Could you check a few things on this model? Use its own coordinates, in mm. Coordinates: 2 decimals unless noted, no trailing zeros.
from build123d import *

# Parameters (mm, degrees)
SKETCH1_W           = 185.999882
SKETCH1_H           = 74.000106
BOSS_EXTRUDE3_DEPTH = 1.5875
CUT_EXTRUDE3_DEPTH  = 2.54


with BuildPart() as part:
    # Sketch1 → Boss-Extrude3 (new body)
    with BuildSketch(Plane(origin=(0, 0, 0), x_dir=(1, 0, 0), z_dir=(0, 1, 0))):
        Rectangle(SKETCH1_W, SKETCH1_H)
    extrude(amount=BOSS_EXTRUDE3_DEPTH)

    # Sketch4 → Cut-Extrude3 (cut)
    with BuildSketch(Plane(origin=(0, 1.5875, 0), x_dir=(1, 0, 0), z_dir=(0, 1, 0))):
        with BuildLine():
            Line((-33.019999998, 0.499998888), (-38.076346482, 0.499998888))
            ThreePointArc((-38.076346482, 0.499998888), (-69.310342417, -8.5e-08), (-38.076346479, -0.499998888))
            Line((-38.076346479, -0.499998888), (-33.019999997, -0.499998888))
            add(Edge.make_bspline(
                [(-33.019999997, -0.499998888), (-32.54632499, -0.569245934), (-31.586035731, -0.710618844), (-29.370983979, -1.038906843), (-27.495063328, -1.325179383), (-25.000131636, -1.708121039), (-22.872397946, -2.043660099), (-20.526372341, -2.417494507), (-18.312405788, -2.778512003), (-16.022726377, -3.157194229), (-13.776510299, -3.536227287), (-10.945442388, -4.021942901), (-6.433516708, -4.814957325), (-1.356746681, -5.744470681), (4.270229912, -6.82483512), (11.013466622, -8.182339851), (16.620878036, -9.365479808), (22.217465189, -10.603163227), (28.231300592, -11.997433679), (33.11855172, -13.176234287), (37.994608625, -14.399821142), (42.858903514, -15.669688211), (47.285116507, -16.866229097), (51.7005538, -18.102139295), (56.104457025, -19.378378553), (59.947265614, -20.531258809), (63.232966999, -21.545846418), (65.965538205, -22.409292492), (68.147965495, -23.110854225), (70.871921061, -24.001687113), (73.589095471, -24.910758606), (76.029944312, -25.746275579), (78.193394279, -26.501694312), (79.81619039, -27.074902775), (81.432049585, -27.651976873), (83.324431409, -28.337781593), (85.465097243, -29.126327671), (87.359843247, -29.836757063), (88.94155129, -30.437597441), (90.322203412, -30.968739967), (91.291423843, -31.343800626), (92.282484454, -31.731855507), (92.741323404, -31.912151608), (92.964000003, -31.999935633)],
                knots=[0.081631279, 0.081631279, 0.081631279, 0.081631279, 0.081631279, 0.096343802, 0.111056325, 0.125768848, 0.140481371, 0.155193894, 0.169906418, 0.184618941, 0.199331464, 0.214043988, 0.228756511, 0.258181558, 0.31703165, 0.346456696, 0.375881743, 0.434731835, 0.464156881, 0.493581928, 0.534357317, 0.563782355, 0.593207404, 0.622632455, 0.652057492, 0.681482549, 0.710907585, 0.725620111, 0.740332636, 0.755045164, 0.769757692, 0.799182725, 0.813895254, 0.821251518, 0.828607782, 0.843320301, 0.858032821, 0.872745338, 0.887457856, 0.894814124, 0.902170393, 0.909526661, 0.91688293, 0.91688293, 0.91688293, 0.91688293, 0.91688293], degree=4))
            Line((92.964000003, -31.999935633), (94.190773048, -31.999935633))
            Line((94.190773048, -31.999935633), (94.190773048, 31.999935633))
            Line((94.190773048, 31.999935633), (92.964000001, 31.999935633))
            add(Edge.make_bspline(
                [(-33.019999998, 0.499998888), (-32.546324991, 0.569245934), (-31.586035733, 0.710618844), (-29.37098398, 1.038906842), (-27.495063329, 1.325179382), (-25.000131637, 1.708121039), (-22.872397948, 2.043660099), (-20.526372343, 2.417494507), (-18.312405789, 2.778512003), (-16.022726379, 3.157194229), (-13.7765103, 3.536227286), (-10.94544239, 4.021942901), (-6.433516709, 4.814957324), (-1.356746682, 5.744470681), (4.27022991, 6.82483512), (11.01346662, 8.182339851), (16.620878035, 9.365479808), (22.217465188, 10.603163227), (28.231300591, 11.997433679), (33.118551718, 13.176234287), (37.994608623, 14.399821142), (42.858903512, 15.669688211), (47.285116506, 16.866229097), (51.700553798, 18.102139295), (56.104457023, 19.378378554), (59.947265613, 20.531258809), (63.232966997, 21.545846418), (65.965538204, 22.409292493), (68.147965493, 23.110854225), (70.87192106, 24.001687113), (73.58909547, 24.910758606), (76.02994431, 25.746275579), (78.193394278, 26.501694312), (79.816190388, 27.074902775), (81.432049584, 27.651976873), (83.324431408, 28.337781594), (85.465097241, 29.126327672), (87.359843245, 29.836757063), (88.941551288, 30.437597442), (90.322203411, 30.968739967), (91.291423842, 31.343800626), (92.282484452, 31.731855507), (92.741323403, 31.912151608), (92.964000001, 31.999935633)],
                knots=[0.081631279, 0.081631279, 0.081631279, 0.081631279, 0.081631279, 0.096343802, 0.111056325, 0.125768848, 0.140481371, 0.155193894, 0.169906418, 0.184618941, 0.199331464, 0.214043988, 0.228756511, 0.258181558, 0.31703165, 0.346456696, 0.375881743, 0.434731835, 0.464156881, 0.493581928, 0.534357317, 0.563782355, 0.593207404, 0.622632455, 0.652057492, 0.681482549, 0.710907585, 0.725620111, 0.740332636, 0.755045164, 0.769757692, 0.799182725, 0.813895254, 0.821251518, 0.828607782, 0.843320301, 0.858032821, 0.872745338, 0.887457856, 0.894814124, 0.902170393, 0.909526661, 0.91688293, 0.91688293, 0.91688293, 0.91688293, 0.91688293], degree=4))
        make_face()
    extrude(amount=-CUT_EXTRUDE3_DEPTH, mode=Mode.SUBTRACT)


solid = part.part
(1) I need wall thicknesses on probe 1 along Z at (x, y) = (55, 1.35); probe 2 along Z at (x, y) = (-63, 0.1). Which ranges of each line are inside material? Lowest first, please.
Answers:
probe 1: z = -37 to -19.06, 19.06 to 37
probe 2: z = -37 to -12.54, 12.54 to 37
(2) We'd pull the mould along X, two halves only. Please class faces 1 (the face through (-22, 0, -9)), 2 (the face through (-69.296, 0.805, -0.68)): +X half, -X half, draft (parallel to the pull), parting line (faces both ways), or undercut.
Answers:
face 1: draft
face 2: undercut
(3) For pin 1 (6 mm diameter, centred on x = -68, z = -17, fed in from -Y), with a flat end and sliding along its axis, tell me the tip position at first contact or that it passes through.
Answers:
pin 1: stops at y = 0
